Read the model definition and answer for the solid it produces. Units are mm, in the model's axes. A direction names the side the tool comes from. Coordinates: 2 decimals unless noted, no trailing zeros. Order: outer loops, then holes, each group sorted by start corner. A loop starts at its lowest first (then second) coordinate and runs counter-clockwise, first axis right, second up. Notation, with made-up numbers: M 41,-39.75 L 93,-39.75 A22 ccw 93,-3.75 Z; hole C 75.25,-19 d2. An arc over 180 degrees is marked long. One line per question, with ' | ' between items. Start each with the question number.
1) Find section B-B, the plane z = 23.55. Write down the section's boundary in (x, y) (3 decimals), plus the area to 3 significant figures.
2) The mould has two halves that part along X. Classify faces 4 (the face through (-13.517, 1.972, 15.24)), 5 (the face through (0, 4, 0)), 6 (the face through (-27.723, 2.028, 13.355)), 7 (the face through (27.72, 1.97, 27.77)): +X half, -X half, draft (parallel to the pull), parting line (faces both ways), or undercut.
3) Find section C-C, the plane y = 2. Count the separate pieces of the cut face and the enclosed holes in it, plus the area to 3 significant figures.
4) A tool of negligible diameter and unlimited length cuts with its end or side. For faces 1 (the face through (-27.77, 2.03, -13.4)), 2 (the face through (-18, 0, 20)), 3 (the face through (17.483, 1.972, -15.76)), from which of +Z, -Z, +X, -X, +Y, -Y can it reach the whole face along a straight path? Write none if from no direction.
5) Given P1, Ø19.5, axis at x = 11, z = -2.5, coming from the -Y side; P2, Ø1.1, axis at x = 0.5, z = -3, coming from the +Y side; P3, Ø1.2, axis at y = 1, z = 0, coming from the -X side (3 decimals); P4, Ø0.5, axis at x = 15, z = 0, coming from the +Y side, each flat-ended and moving along its own axis, determine where each tip first touches the part or whether it passes through.
6) Find section D-D, the plane x = -23.55. Write down the section's boundary in (y, z) (3 decimals).
7) Consider probe 1 along X at (y, z) = (1.6, 15.5) (3 decimals); probe 2 along X at (y, z) = (0.9, 23.55) (3 decimals); probe 3 along Z at (x, y) = (-1, 3.75) (3 decimals). Determine where each line is inside the solid, lowest interval first.
8) Find section A-A, the plane x = -15.5. Write down the section's boundary in (y, z) (3 decimals), plus the area to 3 significant figures.
from build123d import *

# Parameters (mm, degrees)
SKETCH1_R           = 2
SKETCH1_R_2         = 2.5
BOSS_EXTRUDE1_DEPTH = 4
SKETCH2_W           = 1
SKETCH2_H           = 25
CUT_EXTRUDE1_DEPTH  = 1
SKETCH3_W           = 22
SKETCH3_H           = 25
CUT_EXTRUDE2_DEPTH  = 41.679002569
BOSS_EXTRUDE2_REACH = 66.132
FILLET1_R           = 3


with BuildPart() as part:
    # Sketch1 → Boss-Extrude1 (new body)
    with BuildSketch(Plane(origin=(0, 0, 0), x_dir=(1, 0, 0), z_dir=(0, 1, 0))):
        with BuildLine():
            Line((25.625, 28.625), (-25.625, 28.625))
            ThreePointArc((-25.625, 28.625), (-27.746320344, 27.746320344), (-28.625, 25.625))
            Line((-28.625, 25.625), (-28.625, -25.625))
            ThreePointArc((-28.625, -25.625), (-27.746320344, -27.746320344), (-25.625, -28.625))
            Line((-25.625, -28.625), (25.625, -28.625))
            ThreePointArc((25.625, -28.625), (27.746320344, -27.746320344), (28.625, -25.625))
            Line((28.625, -25.625), (28.625, 25.625))
            ThreePointArc((28.625, 25.625), (27.746320344, 27.746320344), (25.625, 28.625))
        make_face()
        with Locations(Location((-15.5, 15.5, 0), (0, 0, 270))):
            Circle(SKETCH1_R, mode=Mode.SUBTRACT)
        with Locations(Location((-23.55, 23.55, 0), (0, 0, 270))):
            Circle(SKETCH1_R_2, mode=Mode.SUBTRACT)
        with Locations(Location((23.55, 23.55, 0), (0, 0, 270))):
            Circle(SKETCH1_R_2, mode=Mode.SUBTRACT)
        with Locations(Location((15.5, 15.5, 0), (0, 0, 270))):
            Circle(SKETCH1_R, mode=Mode.SUBTRACT)
        with Locations(Location((15.5, -15.5, 0), (0, 0, 270))):
            Circle(SKETCH1_R, mode=Mode.SUBTRACT)
        with Locations(Location((-15.5, -15.5, 0), (0, 0, 270))):
            Circle(SKETCH1_R, mode=Mode.SUBTRACT)
        with Locations(Location((-23.55, -23.55, 0), (0, 0, 270))):
            Circle(SKETCH1_R_2, mode=Mode.SUBTRACT)
        with Locations(Location((23.55, -23.55, 0), (0, 0, 270))):
            Circle(SKETCH1_R_2, mode=Mode.SUBTRACT)
    extrude(amount=BOSS_EXTRUDE1_DEPTH)

    # Sketch2 → Cut-Extrude1 (cut)
    with BuildSketch(Plane(origin=(0, 4, 0), x_dir=(1, 0, 0), z_dir=(0, 1, 0))):
        with Locations((-27.125, 0)):
            Rectangle(SKETCH2_W, SKETCH2_H)
        with Locations((-25.125, 0)):
            Rectangle(SKETCH2_W, SKETCH2_H)
        with Locations((-23.125, 0)):
            Rectangle(SKETCH2_W, SKETCH2_H)
        with Locations((-21.125, 0)):
            Rectangle(SKETCH2_W, SKETCH2_H)
        with Locations((-19.125, 0)):
            Rectangle(SKETCH2_W, SKETCH2_H)
        with Locations((-17.125, 0)):
            Rectangle(SKETCH2_W, SKETCH2_H)
        with Locations((-15.125, 0)):
            Rectangle(SKETCH2_W, SKETCH2_H)
        with Locations((-13.125, 0)):
            Rectangle(SKETCH2_W, SKETCH2_H)
        with Locations((-11.125, 0)):
            Rectangle(SKETCH2_W, SKETCH2_H)
        with Locations((-9.125, 0)):
            Rectangle(SKETCH2_W, SKETCH2_H)
        with Locations((-7.125, 0)):
            Rectangle(SKETCH2_W, SKETCH2_H)
        with Locations((-5.125, 0)):
            Rectangle(SKETCH2_W, SKETCH2_H)
        with Locations((-3.125, 0)):
            Rectangle(SKETCH2_W, SKETCH2_H)
        with Locations((-1.125, 0)):
            Rectangle(SKETCH2_W, SKETCH2_H)
        with Locations((0.875, 0)):
            Rectangle(SKETCH2_W, SKETCH2_H)
        with Locations((2.875, 0)):
            Rectangle(SKETCH2_W, SKETCH2_H)
        with Locations((4.875, 0)):
            Rectangle(SKETCH2_W, SKETCH2_H)
        with Locations((6.875, 0)):
            Rectangle(SKETCH2_W, SKETCH2_H)
        with Locations((8.875, 0)):
            Rectangle(SKETCH2_W, SKETCH2_H)
        with Locations((10.875, 0)):
            Rectangle(SKETCH2_W, SKETCH2_H)
        with Locations((12.875, 0)):
            Rectangle(SKETCH2_W, SKETCH2_H)
        with Locations((14.875, 0)):
            Rectangle(SKETCH2_W, SKETCH2_H)
        with Locations((16.875, 0)):
            Rectangle(SKETCH2_W, SKETCH2_H)
        with Locations((18.875, 0)):
            Rectangle(SKETCH2_W, SKETCH2_H)
        with Locations((20.875, 0)):
            Rectangle(SKETCH2_W, SKETCH2_H)
        with Locations((22.875, 0)):
            Rectangle(SKETCH2_W, SKETCH2_H)
        with Locations((24.875, 0)):
            Rectangle(SKETCH2_W, SKETCH2_H)
        with Locations((26.875, 0)):
            Rectangle(SKETCH2_W, SKETCH2_H)
    extrude(amount=-CUT_EXTRUDE1_DEPTH, mode=Mode.SUBTRACT)

    # Sketch3 → Cut-Extrude2 (cut, through all)
    with BuildSketch(Plane.XZ):
        with Locations((-17.625, 0)):
            Rectangle(SKETCH3_W, SKETCH3_H)
    extrude(amount=-CUT_EXTRUDE2_DEPTH, mode=Mode.SUBTRACT)

    # Boss-Extrude2: up to this face of the body (flat: up to its plane)
    boss_extrude2_end = Plane(part.part.faces().sort_by_distance((0, 2, 28.625))[0])
    # Sketch4 → Boss-Extrude2 (add, up to the picked face)
    with BuildSketch(Plane(origin=(0, 0, -28.625), x_dir=(-1, 0, 0), z_dir=(0, 0, -1)), mode=Mode.PRIVATE) as boss_extrude2_sk1:
        with BuildLine():
            Line((-4.249281585, 0), (6.625, 0))
            ThreePointArc((6.625, 0), (1.187859207, -2.75), (-4.249281585, 0))
        make_face()
    boss_extrude2_tool1 = split(extrude(boss_extrude2_sk1.sketch, amount=-BOSS_EXTRUDE2_REACH, mode=Mode.PRIVATE), bisect_by=boss_extrude2_end, keep=Keep.BOTH, mode=Mode.PRIVATE)
    add(boss_extrude2_tool1.solids().sort_by(Axis((-1.187859, -1.121798, -28.625), (0, 0, 1)))[0])

    # Fillet1
    fillet1_edges = [part.edges().sort_by_distance(p)[0] for p in [
        (-28.625, 2, 12.5),
        (-28.625, 2, -12.5),
    ]]
    fillet(fillet1_edges, radius=FILLET1_R)


solid = part.part
Report:
1) outline: M -28.625,0 L -26.05,0 L -26.05,4 L -28.625,4 Z; M -21.05,0 L -6.625,0 A6.75 ccw 4.249,0 L 21.05,0 L 21.05,4 L -21.05,4 Z; M 26.05,0 L 28.625,0 L 28.625,4 L 26.05,4 Z | area: 210 mm^2
2) face 4: undercut | face 5: draft | face 6: -X half | face 7: +X half
3) separate pieces: 1 | enclosed holes: 8 | area: 2,590 mm^2
4) face 1: -X, +Y, -Y | face 2: +Z, -Z, -X, -Y | face 3: +Y, -Y
5) P1: stops at y = -2.29 | P2: stops at y = 4 | P3: stops at x = -6.625 | P4: stops at y = 3
6) outline: M 0,-28.625 L 4,-28.625 L 4,-26.05 L 0,-26.05 Z; M 0,-21.05 L 4,-21.05 L 4,-12.5 L 0,-12.5 Z; M 0,12.5 L 4,12.5 L 4,21.05 L 0,21.05 Z; M 0,26.05 L 4,26.05 L 4,28.625 L 0,28.625 Z
7) probe 1: x = -28.625 to -17.5, -13.5 to 13.5, 17.5 to 28.625 | probe 2: x = -28.625 to -26.05, -21.05 to 21.05, 26.05 to 28.625 | probe 3: z = -28.625 to -12.5, 12.5 to 28.625
8) outline: M 0,-28.625 L 4,-28.625 L 4,-17.5 L 0,-17.5 Z; M 0,-13.5 L 4,-13.5 L 4,-12.5 L 0,-12.5 Z; M 0,12.5 L 4,12.5 L 4,13.5 L 0,13.5 Z; M 0,17.5 L 4,17.5 L 4,28.625 L 0,28.625 Z | area: 97.0 mm^2
